from build123d import *

# Parameters (mm, degrees)
ESQUISSE1_W                  = 80
ESQUISSE1_H                  = 10
ESQUISSE3_R                  = 10
ENL_V_MAT_EXTRU_1_DEPTH      = 476.280969533
R_P_TITION_CIRCULAIRE1_COUNT = 20
BOSS_EXTRU_1_START           = -10
BOSS_EXTRU_1_DEPTH           = 10
BOSS_EXTRU_2_START           = -10
BOSS_EXTRU_2_DEPTH           = 10
BOSS_EXTRU_3_START           = 100
BOSS_EXTRU_3_DEPTH           = 100
ESQUISSE8_W                  = 133.349416634
ESQUISSE8_H                  = 90
ENL_V_MAT_EXTRU_2_DEPTH      = 857.817874815


with BuildPart() as part:
    # Esquisse1 → Révolution1 (revolve)
    with BuildSketch(Plane.XY, mode=Mode.PRIVATE) as r_volution1_sk:
        with Locations((296, 5)):
            Rectangle(ESQUISSE1_W, ESQUISSE1_H)
    revolve(r_volution1_sk.sketch.rotate(Axis((0, 0, 0), (0, 1, 0)), 90), axis=Axis((0, 0, 0), (0, 1, 0)))

    # Esquisse3 → Enlèv. mat.-Extru.1 (cut, through all)
    with BuildSketch(Plane(origin=(0, 10, 0), x_dir=(1, 0, 0), z_dir=(0, 1, 0))):
        with Locations(Location((296, 0, 0), (0, 0, 270))):
            Circle(ESQUISSE3_R)
    enl_v_mat_extru_1 = extrude(amount=-ENL_V_MAT_EXTRU_1_DEPTH, mode=Mode.SUBTRACT)

    # Répétition circulaire1: Enlèv. mat.-Extru.1 ×20 about axis
    r_p_tition_circulaire1_axis = Axis((0, 0, 0), (0, 1, 0))
    for i in range(1, R_P_TITION_CIRCULAIRE1_COUNT):
        add(enl_v_mat_extru_1.rotate(r_p_tition_circulaire1_axis, i * 360 / R_P_TITION_CIRCULAIRE1_COUNT), mode=Mode.SUBTRACT)

    # Esquisse4 → Boss.-Extru.1 (add)
    with BuildSketch(Plane.XZ.offset(BOSS_EXTRU_1_START)):
        with BuildLine():
            Line((516.151015307, -240), (516.151015307, 240))
            Line((516.151015307, 240), (235.151015307, 240))
            ThreePointArc((235.151015307, 240), (336, 0), (235.151015307, -240))
            Line((235.151015307, -240), (516.151015307, -240))
        make_face()
    extrude(amount=BOSS_EXTRU_1_DEPTH)

    # Esquisse5 → Boss.-Extru.2 (add)
    with BuildSketch(Plane.XZ.offset(BOSS_EXTRU_2_START)):
        with BuildLine():
            Line((235.151015307, -240), (362.801598673, -240))
            ThreePointArc((362.801598673, -240), (-435, 0), (362.801598673, 240))
            Line((362.801598673, 240), (235.151015307, 240))
            ThreePointArc((235.151015307, 240), (-336, 0), (235.151015307, -240))
        make_face()
    extrude(amount=BOSS_EXTRU_2_DEPTH)

    # Esquisse6 → Boss.-Extru.3 (add)
    with BuildSketch(Plane(origin=(0, 10, 0), x_dir=(1, 0, 0), z_dir=(0, 1, 0)).offset(BOSS_EXTRU_3_START)):
        with BuildLine():
            Line((516.151015307, 240), (362.801598673, 240))
            ThreePointArc((362.801598673, 240), (-435, 0), (362.801598673, -240))
            Line((362.801598673, -240), (516.151015307, -240))
            Line((516.151015307, -240), (516.151015307, 240))
        make_face()
        with BuildLine():
            ThreePointArc((359.562233834, 234), (-429, 0), (359.562233834, -234))
            Line((359.562233834, -234), (510.151015307, -234))
            Line((510.151015307, -234), (510.151015307, 234))
            Line((510.151015307, 234), (359.562233834, 234))
        make_face(mode=Mode.SUBTRACT)
    extrude(amount=-BOSS_EXTRU_3_DEPTH)

    # Esquisse8 → Enlèv. mat.-Extru.2 (cut, through all)
    with BuildSketch(Plane.XY.offset(240)):
        with Locations((439.47630699, 55)):
            Rectangle(ESQUISSE8_W, ESQUISSE8_H)
    extrude(amount=-ENL_V_MAT_EXTRU_2_DEPTH, mode=Mode.SUBTRACT)


solid = part.part
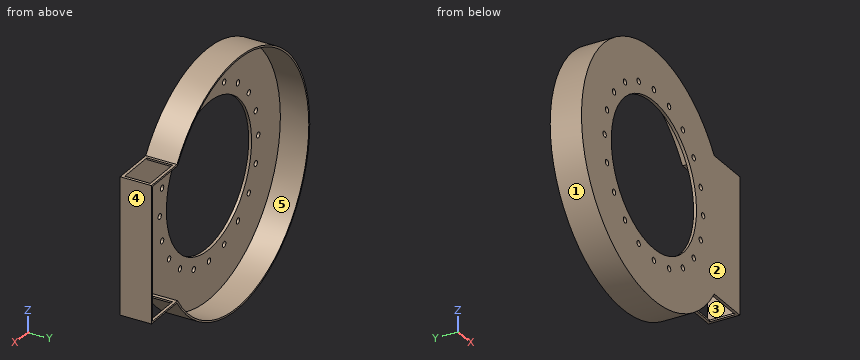
Geometry check sheet. Reference: the model listing, model coordinates, mm. Face numbers are marked on the shaded views. A direction names the side the tool comes from. Coordinates: 2 decimals unless noted, no trailing zeros. Order: outer loops, then holes, each group sorted by start corner. A loop starts at its lowest first (then second) coordinate and runs counter-clockwise, first axis right, second up. Notation, with made-up numbers: M 23,1.5 L 54,1.5 A28 ccw 54,37.5 Z; hole C 84.25,80 d1. An arc over 180 degrees is marked long. Use CSV: the item, a comma, the result in double quotes.
Item 1: Gauge pin test, flat ends, axial feed: pin 1 Ø8 at (x, y) = (-321.5, 53) entering from +Z; pin 2 Ø6 at (x, y) = (-93, 23) entering from +Z; pin 3 Ø12 at (x, z) = (-331.5, -101) entering from +Y; pin 4 Ø18 at (x, z) = (91.47, -281.51) entering from -Y. Record the tip position at first contact, or that the pin passes through.
Returned:
pin 1,"stops at z = 297.35"
pin 2,"stops at z = 425.59"
pin 3,"stops at y = 10"
pin 4,"passes through"
Item 2: Cross-section at D-D on z = -364. Record the cut outline in (x, y), then the cut area to 3 significant figures.
Returned:
outline,"M -238.18,0 L 238.18,0 L 238.18,110 L 227.04,110 L 227.04,10 L -227.04,10 L -227.04,110 L -238.18,110 Z"
area,"6,990 mm2"
Item 3: Tool access check on the marked faces 4 and 5. Record the directions out of +Z, -Z, +X, -X, +Y, -Y that give a thin tool (end or side, any length) a straight path to the whole face; none if there is none.
Returned:
face 4,"+Z, -Z, +X, +Y, -Y"
face 5,"+Y"
Item 4: Cross-section at A-A on y = 71.5. Record the cut outline in (x, z).
Returned:
outline,"M 359.56,-234 A429 cw long 359.56,234 L 372.8,234 L 372.8,240 L 362.8,240 A435 ccw long 362.8,-240 L 372.8,-240 L 372.8,-234 Z; M 506.15,-240 L 516.15,-240 L 516.15,240 L 506.15,240 L 506.15,234 L 510.15,234 L 510.15,-234 L 506.15,-234 Z"
Item 5: Mould release check, pull along Z, two halves, no side actions. Record for the marked faces 1, 2 and 3: pulls with the +Z half, pulls with the -Z half, needs draft (parallel to the pull), parting line crosses it, or undercut.
Returned:
face 1,"parting line crosses it"
face 2,"needs draft"
face 3,"undercut"
Item 6: Cross-section at C-C on z = 204.5. Record the cut outline in (x, y), then the cut area to 3 significant figures.
Returned:
outline,"M -383.93,0 L -154,0 L -154,10 L -377.12,10 L -377.12,110 L -383.93,110 Z; M 154,0 L 516.15,0 L 516.15,110 L 510.15,110 L 510.15,10 L 154,10 Z"
area,"7,200 mm2"
Item 7: Cross-section at B-B on x = -24. Record the cut outline in (y, z), then the cut area to 3 significant figures.
Returned:
outline,"M 0,-434.34 L 110,-434.34 L 110,-428.33 L 10,-428.33 L 10,-254.87 L 0,-254.87 Z; M 0,254.87 L 10,254.87 L 10,428.33 L 110,428.33 L 110,434.34 L 0,434.34 Z"
area,"4,790 mm2"
Item 8: Thickness scan on line 1 along X through (y, z) = (6.25, 0); line 2 along Z through (x, y) = (364, 54.5); line 3 along Y through (x, z) = (-364.5, 11.5). Record the ranges inside material, lowest first.
Returned:
line 1,"x = -435 to -306, -286 to -256, 256 to 286, 306 to 516.15"
line 2,"z = -240 to -234, 234 to 240"
line 3,"y = 0 to 10"
